from build123d import *

# Parameters (mm, degrees)
SKETCH1_W           = 80
SKETCH1_H           = 100
BOSS_EXTRUDE1_DEPTH = 15
SKETCH3_R           = 90
BOSS_EXTRUDE2_DEPTH = 10
SKETCH2_R           = 6
BOSS_EXTRUDE3_DEPTH = 10
SKETCH4_R           = 5
BOSS_EXTRUDE4_DEPTH = 10


with BuildPart() as part:
    # Sketch1 → Boss-Extrude1 (new body)
    with BuildSketch(Plane(origin=(0, 0, 0), x_dir=(0, 0, -1), z_dir=(1, 0, 0))):
        Polygon((40, -20), (40, -50), (80, -50), align=None)
        Rectangle(SKETCH1_W, SKETCH1_H)
        Polygon((-80, -50), (-40, -50), (-40, -20), align=None)
    extrude(amount=BOSS_EXTRUDE1_DEPTH)

    # Sketch3 → Boss-Extrude2 (add)
    with BuildSketch(Plane.XZ.offset(50)):
        with Locations((17.5, 0)):
            Circle(SKETCH3_R)
    extrude(amount=BOSS_EXTRUDE2_DEPTH)

    # Sketch2 → Boss-Extrude3 (add)
    with BuildSketch(Plane(origin=(15, 0, 0), x_dir=(0, 0, -1), z_dir=(1, 0, 0))):
        with Locations((0, 15.728916746)):
            Circle(SKETCH2_R)
    extrude(amount=BOSS_EXTRUDE3_DEPTH)

    # Sketch4 → Boss-Extrude4 (add)
    with BuildSketch(Plane.XZ.offset(60)):
        with Locations((17.5, 0)):
            Circle(SKETCH4_R)
    extrude(amount=BOSS_EXTRUDE4_DEPTH)


solid = part.part
Check sheet for the modelled part. Datum: model origin and axes. Units: mm. A direction names the side the tool comes from. Coordinates: 2 decimals unless noted, no trailing zeros. Write each loop counter-clockwise with the first axis right and the second up, starting at its lowest first coordinate (ties: lowest second). Pieces come first, ordered by that corner, then holes.
Item 1: Cross-section at B-B on z = 0. Record the boundary of the cut face in (x, y), then the cut area to 3 significant figures.
Numbers:
outline: (-72.5, -60) - (12.5, -60) - (12.5, -70) - (22.5, -70) - (22.5, -60) - (107.5, -60) - (107.5, -50) - (15, -50) - (15, 9.73) - (25, 9.73) - (25, 21.73) - (15, 21.73) - (15, 50) - (0, 50) - (0, -50) - (-72.5, -50) - close
area: 3,520 mm2
Item 2: Cross-section at D-D on z = -61.5. Record the boundary of the cut face in (x, y) (3 decimals).
Numbers:
outline: (-48.21, -60) - (83.21, -60) - (83.21, -50) - (15, -50) - (15, -36.125) - (0, -36.125) - (0, -50) - (-48.21, -50) - close
Item 3: Cross-section at A-A on x = 17.5. Record the boundary of the cut face in (y, z).
Numbers:
outline: (-70, -5) - (-60, -5) - (-60, -90) - (-50, -90) - (-50, 90) - (-60, 90) - (-60, 5) - (-70, 5) - close; circle Ø12 at (15.73, 0)
Item 4: Mould release check, pull along Y, two halves, no side actions. Record for faces 1 (the face through (19.93, 9.87, 1.3)), 2 (the face through (7, 50, 1)), 3 (the face through (7, 15, 40)): released by +Y, released by -Y, zero draft, split by the parting line, or undercut.
Numbers:
face 1: undercut
face 2: released by +Y
face 3: zero draft
Item 5: Cross-section at C-C on y = -55.5. Record the boundary of the cut face in (x, z).
Numbers:
outline: circle Ø180 at (17.5, 0)
Item 6: Scan lines: probe 1 along X at (y, z) = (-29, 32.5); probe 2 along Y at (x, z) = (59.5, -23); probe 3 along Z at (x, y) = (94, -55). Record each from-to range of solid material in increasing order.
Numbers:
probe 1: x = 0 to 15
probe 2: y = -60 to -50
probe 3: z = -47.41 to 47.41
Item 7: Depth check by flat-ended pin: pin 1 Ø5 at (x, z) = (11, 14.5) entering from -Y; pin 2 Ø10 at (x, y) = (16, -10) entering from -Z; pin 3 Ø2 at (y, z) = (-24.5, 25) entering from -X. Enter the tip coordinate at first touch or a pass-through.
Numbers:
pin 1: stops at y = -60
pin 2: stops at z = -40
pin 3: stops at x = 0
Item 8: Access from +Z, -Z, +X, -X, +Y, -Y to the whole of each face (thin tool, end or side, straight path). Record for faces 4 (the face through (25, 16, 0)), 5 (the face through (0, 1, 1)), 6 (the face through (12.505, -64.93, 0.22)), 7 (the face through (-2.01, -54.93, -87.86)), 8 (the face through (7, 15, -40)).
Numbers:
face 4: +Z, -Z, +X, +Y
face 5: +Z, -Z, -X, +Y
face 6: -Y
face 7: +Y, -Y
face 8: -Z, +X, -X, +Y
